from build123d import *

# Parameters (mm, degrees)
SKETCH1_R           = 11
SKETCH1_R_2         = 4
BOSS_EXTRUDE1_DEPTH = 7
SKETCH2_R           = 8.25
SKETCH2_R_2         = 6.5
CUT_EXTRUDE1_DEPTH  = 0.2
SKETCH3_R           = 8.25
SKETCH3_R_2         = 6.5
CUT_EXTRUDE2_DEPTH  = 0.2
CHAMFER1_SIZE       = 0.2


with BuildPart() as part:
    # Sketch1 → Boss-Extrude1 (new body)
    with BuildSketch(Plane(origin=(0, 0, 0), x_dir=(1, 0, 0), z_dir=(0, 1, 0))):
        Circle(SKETCH1_R)
        Circle(SKETCH1_R_2, mode=Mode.SUBTRACT)
    extrude(amount=BOSS_EXTRUDE1_DEPTH)

    # Sketch2 → Cut-Extrude1 (cut)
    with BuildSketch(Plane(origin=(0, 7, 0), x_dir=(1, 0, 0), z_dir=(0, 1, 0))):
        Circle(SKETCH2_R)
        Circle(SKETCH2_R_2, mode=Mode.SUBTRACT)
    extrude(amount=-CUT_EXTRUDE1_DEPTH, mode=Mode.SUBTRACT)

    # Sketch3 → Cut-Extrude2 (cut)
    with BuildSketch(Plane.XZ):
        Circle(SKETCH3_R)
        Circle(SKETCH3_R_2, mode=Mode.SUBTRACT)
    extrude(amount=-CUT_EXTRUDE2_DEPTH, mode=Mode.SUBTRACT)

    # Chamfer1
    chamfer1_edges = [part.edges().sort_by_distance(p)[0] for p in [
        (-11, 0, 0),
        (-11, 7, 0),
        (-4, 0, 0),
        (-4, 7, 0),
    ]]
    chamfer(chamfer1_edges, length=CHAMFER1_SIZE)


solid = part.part
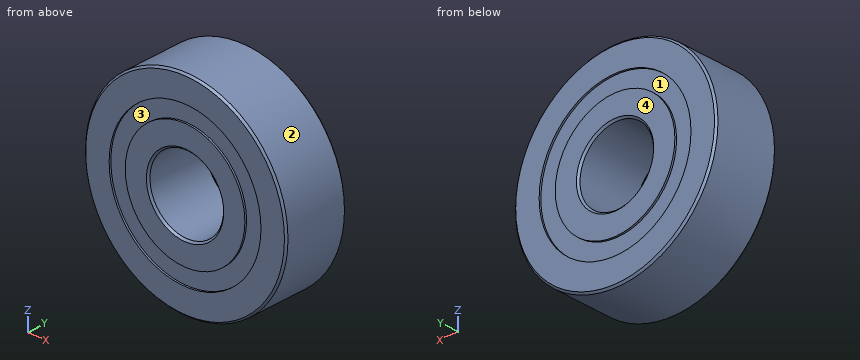
Here's how the part is built. I have some questions about the finished solid (model axes, mm). Face numbers are marked on the shaded views. Coordinates: 2 decimals unless noted, no trailing zeros. Order: outer loops, then holes, each group sorted by start corner. A loop starts at its lowest first (then second) coordinate and runs counter-clockwise, first axis right, second up.
Item 1: I need wall thicknesses on line 1 (X direction, y = 4.5, z = 0); line 2 (Y direction, x = -6.75, z = 4.25); line 3 (Z direction, x = 0.5, y = 6.5). Which ranges of each line are inside material? Lowest first, please.
Result sheet:
line 1: x = -11 to -4, 4 to 11
line 2: y = 0.2 to 6.8
line 3: z = -10.99 to -3.97, 3.97 to 10.99
Item 2: If we mould it in two halves opening along X, with no side actions, what happens to the marked faces 1, 2, 3 and 4? For each: +X half, -X half, draft (parallel to the pull), parting line (faces both ways), or undercut.
Result sheet:
face 1: undercut
face 2: parting line
face 3: undercut
face 4: draft
Item 3: If we section it at C-C on y = 1.5: List the corners of the cut face in (x, z) for me, plus the area to 3 significant figures.
Result sheet:
outline: circle Ø22 at (0, 0); hole circle Ø8 at (0, 0)
area: 330 mm2
Item 4: For P1, Ø1, axis at x = -2, z = 7, coming from the +Y side; P2, Ø1, axis at y = 1.5, z = 2, coming from the -X side, each with a flat end and sliding along its axis, tell me the tip position at first contact or that it passes through.
Result sheet:
P1: stops at y = 6.8
P2: stops at x = -10.9
